Check sheet for the modelled part. Datum: model origin and axes. Units: mm. A direction names the side the tool comes from. Give positions to 0.01 mm unless a question says otherwise; leave off trailing zeros. Write each loop counter-clockwise with the first axis right and the second up, starting at its lowest first coordinate (ties: lowest second). Pieces come first, ordered by that corner, then holes. Notation, with made-up numbers: (52.5, 16.25) -> (80.5, 16.25) arc R8 ccw to (80.5, 24.25) -> close; hole circle Ø2 at (-1.5, 32.25). An arc over 180 degrees is marked (long way). Answer as a JSON object with one key per item and string values.
from build123d import *

# Parameters (mm, degrees)
F1_DEPTH = 25.4


with BuildPart() as f1:
    # F0 (on Front) → F1 (new body, symmetric)
    with BuildSketch(Plane.XZ):
        Polygon((65.332091, 50.400867), (65.332091, 42.799), (65.332091, 28.575), (65.332091, 21.825867), (116.132091, 21.825867), (116.132091, 50.400867), align=None)
        with BuildLine():
            ThreePointArc((60.325, 42.799), (36.796729, 33.053271), (27.051, 9.525))
            Line((27.051, 9.525), (41.275, 9.525))
            ThreePointArc((41.275, 9.525), (46.854616, 22.995384), (60.325, 28.575))
            Line((60.325, 28.575), (65.332091, 28.575))
            Line((65.332091, 28.575), (65.332091, 42.799))
            Line((65.332091, 42.799), (60.325, 42.799))
        make_face()
        Polygon((27.051, 9.525), (-41.275, 9.525), (-41.275, -9.525), (41.275, -9.525), (41.275, 9.525), align=None)
        with BuildLine():
            add(Edge.make_bspline(
                [(-41.275, 9.525), (-13.07586, 35.157815), (15.348731, 53.430766), (60.325, 42.799)],
                knots=[0, 0, 0, 0, 106.909864, 106.909864, 106.909864, 106.909864], degree=3))
            Line((-41.275, 9.525), (27.051, 9.525))
            ThreePointArc((27.051, 9.525), (36.796729, 33.053271), (60.325, 42.799))
        make_face()
    extrude(amount=F1_DEPTH, both=True)


solid = f1.part
1. Access from +Z, -Z, +X, -X, +Y, -Y to the whole of each face (thin tool, end or side, straight path). Record for faces 1 (the face through (65.332, 0, 47)), 2 (the face through (90, 0, 21.826)), 3 (the face through (46.71, -0.36, 22.85)), 4 (the face through (-1, 0, -9.525)).
Determined:
{"face 1": "+Z, +Y, -Y", "face 2": "-Z, +X, +Y, -Y", "face 3": "-Z, +Y, -Y", "face 4": "-Z, +X, -X, +Y, -Y"}
2. Mould release check, pull along X, two halves, no side actions. Record for faces 5 (the face through (-41.275, 0, 0)), 6 (the face through (36, 25.4, 22)), 7 (the face through (65.332, 0, 25)), 8 (the face through (41.275, 0, 0)): released by +X, released by -X, zero draft, split by the parting line, or undercut.
Determined:
{"face 5": "released by -X", "face 6": "zero draft", "face 7": "undercut", "face 8": "released by +X"}
3. Scan lines: L1, parallel to Z at x = 101, y = -4.5; L2, parallel to X at y = 12.5, z = -2.5 (3 decimals); L3, parallel to Z at x = 61, y = -13 (3 decimals). Record each from-to range of solid material in increasing order. Write a range as [from, to].
Determined:
{"L1": "[21.83, 50.4]", "L2": "[-41.275, 41.275]", "L3": "[28.575, 42.799]"}
4. Sectioned sample at B-B, the plane z = -3. Enter the section's corners in (x, y) (3 decimals), plus the area to 3 significant figures.
Determined:
{"outline": "(-41.275, -25.4) -> (41.275, -25.4) -> (41.275, 25.4) -> (-41.275, 25.4) -> close", "area": "4,190 mm^2"}
5. Go/stop test with flat-tipped pins: P1, Ø2, axis at y = -5.5, z = 25.5, coming from the -X side; P2, Ø1.5, axis at x = 64, y = 1.5, coming from the +Z side; P3, Ø1, axis at x = 93.5, y = -2.5, coming from the -Z side. Record where each tip stops, or that it passes through.
Determined:
{"P1": "x = -23.33", "P2": "z = 42.8", "P3": "z = 21.83"}
6. Sectioned sample at A-A, the plane x = 98.5. Enter the section's corners in (y, z), plus the area to 3 significant figures.
Determined:
{"outline": "(-25.4, 21.83) -> (25.4, 21.83) -> (25.4, 50.4) -> (-25.4, 50.4) -> close", "area": "1,450 mm^2"}
